Verification items for the finished model (mm, model axes). Face numbers are marked on the shaded views. A direction names the side the tool comes from. Coordinates: 2 decimals unless noted, no trailing zeros. Write each loop counter-clockwise with the first axis right and the second up, starting at its lowest first coordinate (ties: lowest second). Pieces come first, ordered by that corner, then holes. Notation, with made-up numbers: (26.5, 63.5) -> (67.5, 63.5) arc R30 ccw to (67.5, 97.5) -> close; hole circle Ø8 at (81.5, 88.25). An arc over 180 degrees is marked (long way). Write item = value, one per line. Start each with the question number.
(1) Gauge pin test, flat ends, axial feed: pin 1 Ø5 at (x, z) = (36.195, 31.75) entering from +Y; pin 2 Ø8 at (y, z) = (13, 20.5) entering from -X (3 decimals); pin 3 Ø10 at (x, z) = (36.195, -31.75) entering from +Y; pin 4 Ø4 at (x, z) = (33, -29.5) entering from -Y. Record the tip position at first contact, or that the pin passes through.
(2) Section check A-A (z = 31.75). Record the cut outline in (x, y) (3 decimals).
(3) Section check D-D (y = 26). Record the cut outline in (x, z) (3 decimals).
(4) Set-up check for the marked faces 1 and 2: record each of +Z, -Z, +X, -X, +Y, -Y from which the full face is reachable in a straight line by a thin tool's end or side.
(5) Section check B-B (x = -18). Record the cut outline in (y, z) (3 decimals).
(6) Material ranges on probe 1 along Z at (x, y) = (-1.5, 4.5) (3 decimals); probe 2 along X at (y, z) = (-1.5, -31.75) (3 decimals); probe 3 along Z at (x, y) = (-38.5, -11) (3 decimals), recorded low to high. Write a range as [from, to].
(7) Section check C-C (y = 10). Record the cut outline in (x, z) (3 decimals), plus the area to 3 significant figures.
(8) Mould release check, pull along Z, two halves, no side actions. Record for the marked faces 3, 4, 5 and 6: released by +Z, released by -Z, zero draft, split by the parting line, or undercut.
Autodesk Inventor part; units mm, degrees
ref_plane "YZ Plane" through (0, 0, 0) normal (1, 0, 0) x (0, 1, 0)
ref_plane "XZ Plane" through (0, 0, 0) normal (0, 1, 0) x (-1, 0, 0)
ref_plane "XY Plane" through (0, 0, 0) normal (0, 0, 1) x (1, 0, 0)
sketch "Sketch1" plane through (0, 0, 0) normal (0, 1, 0) x (-1, 0, 0)
  line L0 (42.545, 67.945) -> (-42.545, 67.945)
  line L1 (-42.545, -67.945) -> (42.545, -67.945)
  line L2 (42.545, 67.945) -> (-42.545, -67.945) construction
  line L3 (-42.545, 67.945) -> (42.545, -67.945) construction
  line L4 (42.545, 60.325) -> (-1.905, 60.325)
  line L5 (-1.905, 60.325) -> (-1.905, 41.275)
  line L6 (36.0369, 0) -> (-87.2324, 0)
  line L7 (42.545, -60.325) -> (-1.905, -60.325)
  line L8 (-1.905, -60.325) -> (-1.905, -41.275)
  line L9 (-1.905, -41.275) -> (4.445, -41.275)
  line L10 (4.445, 41.275) -> (4.445, -41.275)
  line L11 (-1.905, 41.275) -> (4.445, 41.275)
  line L12 (42.545, -67.945) -> (42.545, -60.325)
  line L13 (42.545, 60.325) -> (42.545, 67.945)
  arc A0 (-42.545, -13.97) -> (-42.545, 13.97) centre (-42.545, 0) ccw
  line L14 (-42.545, 67.945) -> (-42.545, 13.97)
  line L15 (-42.545, -13.97) -> (-42.545, -67.945)
  point P0 (0, 0)
  dimension "d0" = 85.09
  dimension "d2" = 7.62
  dimension "d4" = 19.05
  dimension "d5" = 7.62
  dimension "d6" = 6.35
  dimension "d7" = 135.89
  dimension "d8" = 44.45
  dimension "d9" = 27.94
  dimension "d10" = 53.975
  dimension "d11" = 53.975
extrude "Extrusion1" add sketch "Sketch1" along normal mid plane 60.96
sketch "Sketch2" plane through (0, 30.48, 0) normal (0, 1, 0) x (1, 0, 0)
  arc A0 (36.195, -25.273) -> (36.195, -38.227) centre (36.195, -31.75) ccw
  line L0 (36.195, -38.227) -> (42.545, -38.227)
  line L1 (36.195, -25.273) -> (42.545, -25.273)
  line L2 (42.545, 13.97) -> (42.545, 67.945)
  line L3 (42.545, -38.227) -> (42.545, -25.273)
  line L4 (42.545, -67.945) -> (42.545, -13.97)
  line L5 (-51.5832, 0) -> (64.091, 0)
  line L6 (-42.545, -67.945) -> (42.545, -67.945)
  arc A1 (36.195, 38.227) -> (36.195, 25.273) centre (36.195, 31.75) ccw
  line L7 (36.195, 38.227) -> (42.545, 38.227)
  line L8 (36.195, 25.273) -> (42.545, 25.273)
  line L9 (42.545, 38.227) -> (42.545, 25.273)
  point P0 (0, 0)
  point P1 (36.195, 47.3075)
  point P2 (36.195, 34.6075)
  point P3 (42.545, 25.273)
  dimension "d15" = 12.954
  dimension "d23" = 67.945
  dimension "d24" = 63.5
  dimension "d25" = 6.35
  dimension "d26" = 12.954
extrude "Extrusion2" cut sketch "Sketch2" against normal blind 6.35
mirror "Mirror1" about plane through (0, 0, 0) normal (0, 1, 0) of "Extrusion2"
sketch "Sketch3" plane through (0, 24.13, 0) normal (0, 1, 0) x (1, 0, 0)
  arc A0 (36.195, -25.273) -> (36.195, -38.227) centre (36.195, -31.75) ccw
  circle A1 centre (36.195, -31.75) radius 3.175
  line L0 (-42.9578, 0) -> (76.8761, 0)
  circle A2 centre (36.195, 31.75) radius 3.175
  point P0 (0, 0)
  dimension "d19" = 6.35
extrude "Extrusion3" cut sketch "Sketch3" against normal through all
sketch "Sketch4" plane through (-42.545, 30.48, 67.945) normal (0, 0, 1) x (1, 0, 0)
  point P0 (42.545, -30.48)
properties part number "Relaxation chamber holder"
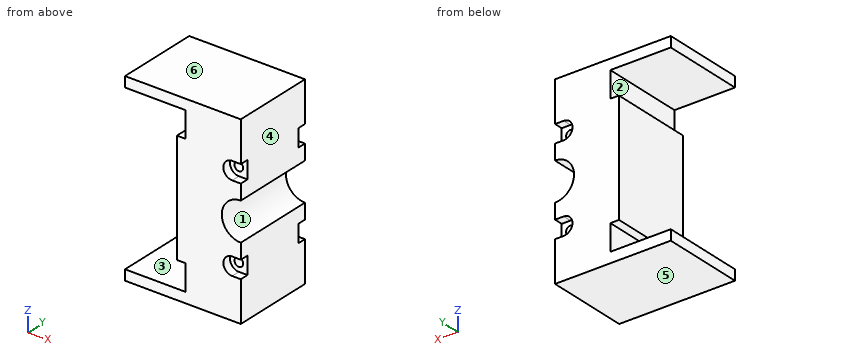
Response:
q1.pin_1 = through
q1.pin_2 = -4.445
q1.pin_3 = 24.13
q1.pin_4 = -24.13
q2.outline = (-4.445, -30.48) -> (29.718, -30.48) -> (29.718, -24.13) -> (33.02, -24.13) -> (33.02, 24.13) -> (29.718, 24.13) -> (29.718, 30.48) -> (-4.445, 30.48) -> close; (39.37, -24.13) -> (42.545, -24.13) -> (42.545, 24.13) -> (39.37, 24.13) -> close
q3.outline = (-42.545, -67.945) -> (42.545, -67.945) -> (42.545, -38.227) -> (36.195, -38.227) arc R6.477 cw to (36.195, -25.273) -> (42.545, -25.273) -> (42.545, -13.97) arc R13.97 cw to (42.545, 13.97) -> (42.545, 25.273) -> (36.195, 25.273) arc R6.477 cw to (36.195, 38.227) -> (42.545, 38.227) -> (42.545, 67.945) -> (-42.545, 67.945) -> (-42.545, 60.325) -> (1.905, 60.325) -> (1.905, 41.275) -> (-4.445, 41.275) -> (-4.445, -41.275) -> (1.905, -41.275) -> (1.905, -60.325) -> (-42.545, -60.325) -> close
q4.face_1 = +X, +Y, -Y
q4.face_2 = -X, +Y, -Y
q5.outline = (-30.48, -67.945) -> (30.48, -67.945) -> (30.48, -60.325) -> (-30.48, -60.325) -> close; (-30.48, 60.325) -> (30.48, 60.325) -> (30.48, 67.945) -> (-30.48, 67.945) -> close
q6.probe_1 = [-67.945, -60.325], [-41.275, 41.275], [60.325, 67.945]
q6.probe_2 = [-4.445, 33.02], [39.37, 42.545]
q6.probe_3 = [-67.945, -60.325], [60.325, 67.945]
q7.outline = (-42.545, -67.945) -> (42.545, -67.945) -> (42.545, -13.97) arc R13.97 cw to (42.545, 13.97) -> (42.545, 67.945) -> (-42.545, 67.945) -> (-42.545, 60.325) -> (1.905, 60.325) -> (1.905, 41.275) -> (-4.445, 41.275) -> (-4.445, -41.275) -> (1.905, -41.275) -> (1.905, -60.325) -> (-42.545, -60.325) -> close; hole circle Ø6.35 at (36.195, -31.75); hole circle Ø6.35 at (36.195, 31.75)
q7.area = 6,350 mm2
q8.face_3 = undercut
q8.face_4 = zero draft
q8.face_5 = released by -Z
q8.face_6 = released by +Z
